Geometry: final body of the model. Coordinates: model frame, mm. Face numbers are marked on the shaded views. Round coordinates to 2 decimals unless told otherwise and drop trailing zeros. Order: outer loops, then holes, each group sorted by start corner. A loop starts at its lowest first (then second) coordinate and runs counter-clockwise, first axis right, second up. Notation, with made-up numbers: M -17,-14.5 L -8,-14.5 A24 ccw -8,3.5 Z; hole C 48.5,43.25 d5. An arc over 180 degrees is marked long. Put each result on its own line as item: value. Start each with the question number.
1) Section D-D, the plane y = 3.5. Return loops of the section in (x, z), then the cut area to 3 significant figures.
2) Draft query along X for the marked faces 1, 2 and 3. Return one class per face: pulls with the +X half, pulls with the -X half, needs draft (parallel to the pull), parting line crosses it, or undercut.
3) First-contact query: P1, Ø2, axis at x = 1, y = 21, coming from the -Z side; P2, Ø1.5, axis at x = -3, y = 10.5, coming from the +Z side; P3, Ø2, axis at x = -2.5, y = 20, coming from the -Z side. Flat tips, straight axial feed; report the tip coordinate or a pass-through.
4) Section B-B, the plane z = 0. Return loops of the section in (x, y), then the cut area to 3 significant figures.
5) Section C-C, the plane y = 9.5. Return loops of the section in (x, z), then the cut area to 3 significant figures.
6) Material intervals for probe 1 along Z at (x, y) = (0, 11.75); probe 2 along Z at (x, y) = (-0.75, 14.5), sorted ascending. Write a range as [from, to].
7) Section A-A, the plane x = 0. Return loops of the section in (y, z), then the cut area to 3 significant figures.
Autodesk Inventor part; units mm, degrees
ref_plane "YZ Plane" through (0, 0, 0) normal (1, 0, 0) x (0, 1, 0)
ref_plane "XZ Plane" through (0, 0, 0) normal (0, 1, 0) x (-1, 0, 0)
ref_plane "XY Plane" through (0, 0, 0) normal (0, 0, 1) x (1, 0, 0)
sketch "Sketch1" plane through (0, 0, 0) normal (0, 1, 0) x (-1, 0, 0)
  circle A0 centre (0, 0) radius 5.15
  dimension "d0" = 10.3
extrude "Extrusion1" add sketch "Sketch1" along normal blind 6
sketch "Sketch2" plane through (0, 6, 0) normal (0, 1, 0) x (1, 0, 0)
  circle A0 centre (0, 0) radius 5.2
  dimension "d3" = 10.4
extrude "Extrusion2" add sketch "Sketch2" along normal blind 20
fillet "Fillet1" radius 0.5 2 edges at (-5.2, 26, 0) (5.15, 0, 0)
sketch "Sketch3" plane through (0, 26, 0) normal (0, 1, 0) x (1, 0, 0)
  circle A0 centre (0, 0) radius 2.5
  dimension "d7" = 5
extrude "Extrusion3" cut sketch "Sketch3" against normal blind 30
properties part number "Schnecke_26mm_5mm"
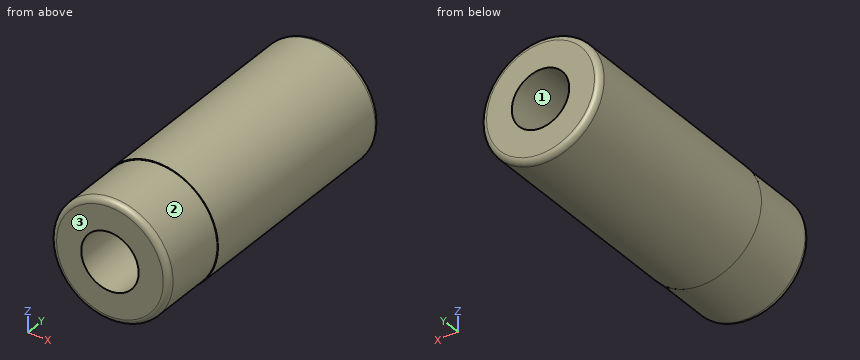
Result sheet:
1. outline: C 0,0 d10.3; hole C 0,0 d5
1. area: 63.7 mm2
2. face 1: undercut
2. face 2: parting line crosses it
2. face 3: needs draft
3. P1: stops at z = -5.2
3. P2: stops at z = 4.69
3. P3: stops at z = -4.98
4. outline: M -5.2,6 L -5.15,6 L -5.15,0.5 A0.5 ccw -4.65,0 L -2.5,0 L -2.5,26 L -4.7,26 A0.5 ccw -5.2,25.5 Z; M 2.5,0 L 4.65,0 A0.5 ccw 5.15,0.5 L 5.15,6 L 5.2,6 L 5.2,25.5 A0.5 ccw 4.7,26 L 2.5,26 Z
4. area: 140 mm2
5. outline: C 0,0 d10.4; hole C 0,0 d5
5. area: 65.3 mm2
6. probe 1: z = [-5.2, -2.5], [2.5, 5.2]
6. probe 2: z = [-5.15, -2.38], [2.38, 5.15]
7. outline: M 0,-4.65 A0.5 ccw 0.5,-5.15 L 6,-5.15 L 6,-5.2 L 25.5,-5.2 A0.5 ccw 26,-4.7 L 26,-2.5 L 0,-2.5 Z; M 0,2.5 L 26,2.5 L 26,4.7 A0.5 ccw 25.5,5.2 L 6,5.2 L 6,5.15 L 0.5,5.15 A0.5 ccw 0,4.65 Z
7. area: 140 mm2
